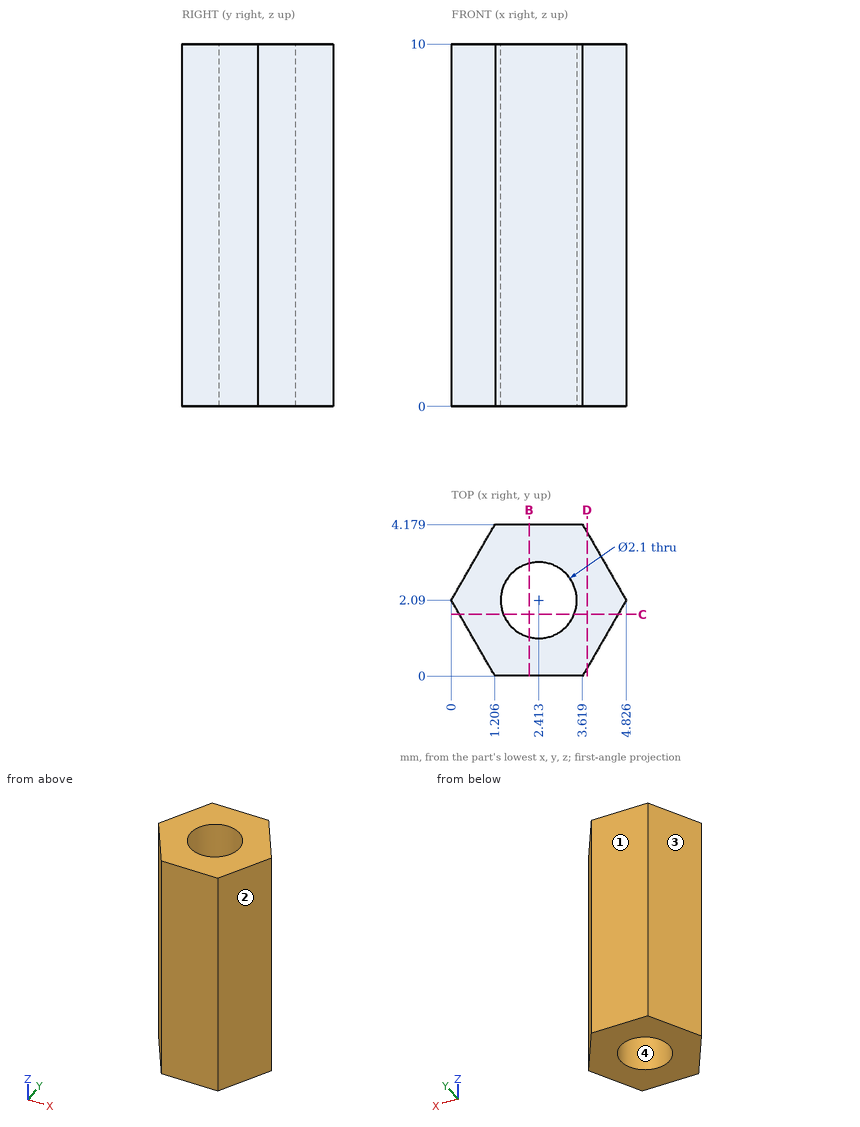
Print and shaded views of the part. All mm, measured from the part's lowest x, y and z. Coordinates: 2 decimals unless noted, no trailing zeros. Write each loop counter-clockwise with the first axis right and the second up, starting at its lowest first coordinate (ties: lowest second). Pieces come first, ordered by that corner, then holes. Notation, with made-up numbers: M 42,6.25 L 73,6.25 A8 cw 73,20.25 Z; hole C -2,86 d6. An arc over 180 degrees is marked long. Return JSON: item names as keys, results as strings.
1. Flat gauge pin, fed straight in: pin 1 Ø2 at (x, y) = (4.5, 1) entering from -Z. Where does the tip first touch, or does it go through?
Determined:
{"pin 1": "z = 0"}
2. Saw through at C-C, the plane y = 1.7. Write the cut outline in (x, z) (1 decimal).
Determined:
{"outline": "M 0.2,0 L 1.4,0 L 1.4,10 L 0.2,10 Z; M 3.4,0 L 4.6,0 L 4.6,10 L 3.4,10 Z"}
3. Pull direction X, two halves, no side cores. Call the marked faces 1, 2, 3 and 4: pulls with the +X half, pulls with the -X half, needs draft (parallel to the pull), parting line crosses it, or undercut.
Determined:
{"face 1": "needs draft", "face 2": "pulls with the +X half", "face 3": "pulls with the -X half", "face 4": "undercut"}
4. Probe L1, parallel to Y at x = 2.65, z = 1; L2, parallel to X at y = 1.85, z = 4 (1 decimal); L3, parallel to Y at x = 3, z = 1.25. List the from-to ranges inside material, lowest first.
Determined:
{"L1": "0 to 1.07, 3.11 to 4.18", "L2": "0.1 to 1.4, 3.4 to 4.7", "L3": "0 to 1.22, 2.96 to 4.18"}
5. Saw through at D-D, the plane x = 3.75. Write the cut outline in (y, z).
Determined:
{"outline": "M 0.23,0 L 3.95,0 L 3.95,10 L 0.23,10 Z"}
6. Saw through at B-B, the plane x = 2.15. Write the cut outline in (y, z).
Determined:
{"outline": "M 0,0 L 1.07,0 L 1.07,10 L 0,10 Z; M 3.11,0 L 4.18,0 L 4.18,10 L 3.11,10 Z"}
